Build history of the part. All positions in model axes, mm. Round coordinates to 2 decimals unless told otherwise and drop trailing zeros. Loops run counter-clockwise (first coordinate to the right, second up) from the corner with the lowest first, then second, coordinate; pieces in that order, holes last. Notation, with made-up numbers: (-16.75, -32) - (-5.75, -32) arc R9 ccw to (-5.75, -25) - close; hole circle Ø10 at (28, 6). An arc over 180 degrees is marked (long way). Use a Markdown table: item, result.
from build123d import *

# Parameters (mm, degrees)
SKETCH1_R               = 2.475
BOSS_EXTRUDE1_DEPTH     = 8
CUT_EXTRUDE1_DEPTH      = 9.732196173
CUT_EXTRUDE1_DEPTH_BACK = 9.732196173
SKETCH2_R               = 1.5
CUT_EXTRUDE3_DEPTH      = 9.732196321
CUT_EXTRUDE3_DEPTH_BACK = 9.732196321
SKETCH5_R               = 4
FILLET1_R               = 0.25


with BuildPart() as part:
    # Sketch1 → Boss-Extrude1 (new, symmetric)
    with BuildSketch(Plane(origin=(0, 0, 0), x_dir=(1, 0, 0), z_dir=(0, 1, 0))):
        with Locations(Location((0, 0, 0), (0, 0, 270))):
            Circle(SKETCH1_R)
    extrude(amount=BOSS_EXTRUDE1_DEPTH, both=True)

    # Sketch2 → Cut-Extrude1 (cut, two sides: drawn at the far end of the back side and taken through both)
    with BuildSketch(Plane.XY.offset(-CUT_EXTRUDE1_DEPTH_BACK)):
        with Locations(Location((0, 0, 0), (0, 0, 89.999999987))):
            Circle(SKETCH2_R)
    extrude(amount=CUT_EXTRUDE1_DEPTH + CUT_EXTRUDE1_DEPTH_BACK, mode=Mode.SUBTRACT)

    # Sketch5 → Cut-Extrude3 (cut, two sides: drawn at the far end of the back side and taken through both)
    with BuildSketch(Plane(origin=(0, 0, 0), x_dir=(0, 0, -1), z_dir=(1, 0, 0)).offset(-CUT_EXTRUDE3_DEPTH_BACK)):
        with Locations((-5.97, 0)):
            Circle(SKETCH5_R)
    extrude(amount=CUT_EXTRUDE3_DEPTH + CUT_EXTRUDE3_DEPTH_BACK, mode=Mode.SUBTRACT)

    # Fillet1
    fillet1_edges = [part.edges().sort_by_distance(p)[0] for p in [
        (0, -8, -2.475),
        (0, 8, -2.475),
    ]]
    fillet(fillet1_edges, radius=FILLET1_R)


solid = part.part
Q1. Pull direction Y, two halves, no side cores. Call faces 1 (the face through (0, 8, 0)), 2 (the face through (0, -8, 0)), 3 (the face through (1.7, 0.1, -1.8)), 4 (the face through (-0.07, -1.5, -0.14)): pulls with the +Y half, pulls with the -Y half, needs draft (parallel to the pull), parting line crosses it, or undercut.
Results found:
| item | result |
|---|---|
| face 1 | pulls with the +Y half |
| face 2 | pulls with the -Y half |
| face 3 | needs draft |
| face 4 | undercut |
Q2. Cut at B-B, the plane z = 0. List the corners of the cut face in (x, y) (3 decimals).
Results found:
| item | result |
|---|---|
| outline | (-2.475, -7.75) arc R0.25 ccw to (-2.225, -8) - (2.225, -8) arc R0.25 ccw to (2.475, -7.75) - (2.475, 7.75) arc R0.25 ccw to (2.225, 8) - (-2.225, 8) arc R0.25 ccw to (-2.475, 7.75) - close; hole circle Ø3 at (0, 0) |
Q3. Probe line 1 (Y direction, x = 0.2, z = -1.75); line 2 (X direction, y = 0, z = 0) (3 decimals); line 3 (X direction, y = 0, z = -1). List the from-to ranges inside material, lowest first.
Results found:
| item | result |
|---|---|
| line 1 | y = -8 to -1.49, 1.49 to 8 |
| line 2 | x = -2.475 to -1.5, 1.5 to 2.475 |
| line 3 | x = -2.26 to -1.5, 1.5 to 2.26 |
Q4. Drop a flat-ended pin along its axis: pin 1 (1.5 mm diameter, centred on y = 2, z = -1, fed in from -X). Give the stop position or say it passes through.
Results found:
| item | result |
|---|---|
| pin 1 | stops at x = -2.46 |
Q5. Cut at D-D, the plane y = -7. List the corners of the cut face in (x, z) (3 decimals), plus the area to 3 significant figures.
Results found:
| item | result |
|---|---|
| outline | circle Ø4.95 at (0, 0) |
| area | 19.2 mm2 |
Q6. Cut at C-C, the plane y = -0.75. List the corners of the cut face in (x, z) (3 decimals).
Results found:
| item | result |
|---|---|
| outline | (-1.4, 2.041) arc R2.475 ccw to (-1.299, -2.107) - (-1.299, 2.041) - close; (1.299, -2.107) arc R2.475 ccw to (1.4, 2.041) - (1.299, 2.041) - close |
